The listing builds one solid part. Answer for the finished solid, in the listing's coordinates (mm). Face numbers are marked on the shaded views. A direction names the side the tool comes from. Give positions to 0.01 mm unless a question says otherwise; leave off trailing zeros. Loops run counter-clockwise (first coordinate to the right, second up) from the corner with the lowest first, then second, coordinate; pieces in that order, holes last. Notation, with made-up numbers: (30.5, -3) - (43.5, -3) arc R23 ccw to (43.5, 26) - close; hole circle Ø7 at (-29, -35.75). An arc over 180 degrees is marked (long way). One line per item, written item: value. Start each with the question number.
from build123d import *

# Parameters (mm, degrees)
F0_W     = 10
F0_H     = 18.5
F2_DEPTH = 10
F3_DEPTH = 3
F0_H_2   = 10
F4_DEPTH = 8
F1_R     = 2
F5_DEPTH = 25
F6_SIZE  = 2.5
F7_R     = 1.99999


# Not quite as in the source:
# - a fillet or chamfer is up to 0.001 mm smaller than in the source, because OpenCascade refuses the exact size


with BuildPart() as f2:
    # F0 (on Top) → F2 (new body)
    with BuildSketch(Plane.XY):
        with Locations((-10.5, 0.1457649022)):
            Rectangle(F0_W, F0_H)
        Polygon((5.5, 17.5), (5.5, 27.5), (-5.5, 27.5), (-5.5, 17.5), (-15.5, 17.5), (-15.5, 9.3957649022), (-5.5, 9.3957649022), (-5.5, -9.1042350978), (-15.5, -9.1042350978), (-15.5, -17.5), (-5.5, -17.5), (-5.5, -27.5), (5.5, -27.5), (5.5, -17.5), (15.5, -17.5), (15.5, 17.5), align=None)
    extrude(amount=F2_DEPTH)

    # F0 (on Top) → F3 (cut)
    with BuildSketch(Plane.XY):
        with Locations((-10.5, 0.1457649022)):
            Rectangle(F0_W, F0_H)
    extrude(amount=F3_DEPTH, mode=Mode.SUBTRACT)

    # F0 (on Top) → F4 (join)
    with BuildSketch(Plane.XY):
        with Locations((-10.5, 22.5)):
            Rectangle(F0_W, F0_H_2)
        with Locations((10.5, 22.5)):
            Rectangle(F0_W, F0_H_2)
        with Locations((-10.5, -22.5)):
            Rectangle(F0_W, F0_H_2)
        with Locations((10.5, -22.5)):
            Rectangle(F0_W, F0_H_2)
    extrude(amount=F4_DEPTH)

    # F1 (on Top) → F5 (cut)
    with BuildSketch(Plane.XY):
        with Locations((-10.4999503866, 22.4999412894)):
            Circle(F1_R)
        with Locations((10.4999503866, 22.4999412894)):
            Circle(F1_R)
        with Locations((-10.4999503866, -22.4999412894)):
            Circle(F1_R)
        with Locations((10.4999503866, -22.4999412894)):
            Circle(F1_R)
    extrude(amount=F5_DEPTH, mode=Mode.SUBTRACT)

    # F6
    f6_edges = [f2.edges().sort_by_distance(p)[0] for p in [
        (-12.49995, 22.499941, 8),
        (8.49995, 22.499941, 8),
        (8.49995, -22.499941, 8),
        (-12.49995, -22.499941, 8),
    ]]
    chamfer(f6_edges, length=F6_SIZE)

    # F7 (radius 2 in the source; OpenCascade refuses exactly that, so slightly less here)
    f7_edges = [f2.edges().sort_by_distance(p)[0] for p in [
        (-10.5, -17.5, 10),
        (-5.5, -22.5, 10),
        (-10.5, 17.5, 10),
        (-5.5, 22.5, 10),
        (5.5, 22.5, 10),
        (10.5, 17.5, 10),
        (10.5, -17.5, 10),
        (5.5, -22.5, 10),
    ]]
    fillet(f7_edges, radius=F7_R)


solid = f2.part
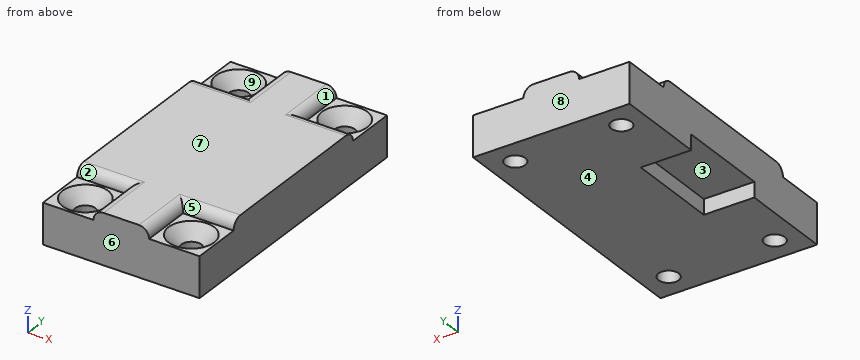
1. For the marked faces 1, 2, 3, 4 and 5, determine the directions among +Z, -Z, +X, -X, +Y, -Y from which every point of the face is accessible in a straight line to the end or side of a thin tool.
2. A cutting plane is placed at A-A (z = 4.75). Determine the outline of the cut face in (x, y).
3. Find the intervals of material crossed by L1, parallel to X at y = 21, z = 3; L2, parallel to Y at x = 11, z = 1.25; L3, parallel to Y at x = -10.5, z = 6, in increasing order. Write a range as [from, to].
4. A cutting plane is placed at B-B (y = 3). Determine the outline of the cut face in (x, z).
5. Flat-ended cylindrical pins translate along their axes: pin 1 (6.5 mm diameter, centred on x = -10.5, y = 22.5, fed in from +Z); pin 2 (3.5 mm diameter, centred on x = 10.5, y = 22.5, fed in from -Z); pin 3 (8 mm diameter, centred on x = -10.5, y = 4.5, fed in from -Z); pin 4 (11 mm diameter, centred on x = 11.5, y = 20, fed in from +Z). Find the tip coordinate at first contact, or state that the pin passes through.
6. Determine the mould class of the marked faces 6, 7, 8 and 9 for opening direction Y: released by +Y, released by -Y, zero draft, split by the parting line, or undercut.
Results below:
1. face 1: +Z, +X, +Y
1. face 2: +Z, -X, -Y
1. face 3: -Z, -X
1. face 4: -Z, +X, -X, +Y, -Y
1. face 5: +Z, +X, -Y
2. outline: (-15.5, -27.5) - (15.5, -27.5) - (15.5, 27.5) - (-15.5, 27.5) - close; hole circle Ø4 at (-10.5, -22.5); hole circle Ø4 at (-10.5, 22.5); hole circle Ø4 at (10.5, -22.5); hole circle Ø4 at (10.5, 22.5)
3. L1: x = [-15.5, -11.82], [-9.18, 9.18], [11.82, 15.5]
3. L2: y = [-27.5, -24.44], [-20.56, 20.56], [24.44, 27.5]
3. L3: y = [-27.5, -25], [-20, 20], [25, 27.5]
4. outline: (-15.5, 3) - (-5.5, 3) - (-5.5, 0) - (15.5, 0) - (15.5, 10) - (-15.5, 10) - close
5. pin 1: stops at z = 6.75
5. pin 2: passes through
5. pin 3: stops at z = 3
5. pin 4: stops at z = 10
6. face 6: released by -Y
6. face 7: zero draft
6. face 8: released by +Y
6. face 9: undercut
